```python
from build123d import *

# Parameters (mm, degrees)
SKETCH_1_R          = 6
EXTRUDE_1_DEPTH     = 5
SKETCH_7_R          = 7
EXTRUDE_6_DEPTH     = 1
EXTRUDE_2_DEPTH     = 13
CUT_EXTRUDE_1_DEPTH = 19


with BuildPart() as part:
    # 草图1 → 凸台-拉伸1 (new body)
    with BuildSketch(Plane.XY):
        Circle(SKETCH_1_R)
    extrude(amount=EXTRUDE_1_DEPTH)

    # 草图7 → 凸台-拉伸6 (add)
    with BuildSketch(Plane.XY.offset(5)):
        Circle(SKETCH_7_R)
    extrude(amount=-EXTRUDE_6_DEPTH)

    # 草图2 → 凸台-拉伸2 (add)
    with BuildSketch(Plane.XY.offset(5)):
        with BuildLine():
            ThreePointArc((4, 0), (1.414213562, 3.741657387), (-3, 2.645751311))
            Line((-3, 2.645751311), (-3, -2.645751311))
            ThreePointArc((-3, -2.645751311), (1.414213562, -3.741657387), (4, 0))
        make_face()
    extrude(amount=EXTRUDE_2_DEPTH)

    # 草图8 → 切除-拉伸1 (cut, through all)
    with BuildSketch(Plane.XY):
        with BuildLine():
            ThreePointArc((2.6, 0), (0.721110255, 2.497999199), (-2.2, 1.385640646))
            Line((-2.2, 1.385640646), (-2.2, -1.385640646))
            ThreePointArc((-2.2, -1.385640646), (0.721110255, -2.497999199), (2.6, 0))
        make_face()
    extrude(amount=CUT_EXTRUDE_1_DEPTH, mode=Mode.SUBTRACT)


solid = part.part
```
Design review of the part built by this model. Coordinates are the model's own, in mm. A direction names the side the tool comes from. Round coordinates to 2 decimals unless told otherwise and drop trailing zeros. Order: outer loops, then holes, each group sorted by start corner. A loop starts at its lowest first (then second) coordinate and runs counter-clockwise, first axis right, second up. Notation, with made-up numbers: (-28.5, 71) - (-19.5, 71) arc R25 ccw to (-19.5, 103) - close; hole circle Ø6 at (15.25, 47). An arc over 180 degrees is marked (long way). Return JSON: item names as keys, results as strings.
Q1. For pin 1 Ø4 at (y, z) = (-2, 14.5) entering from -X; pin 2 Ø1.5 at (y, z) = (-3, 5.5) entering from -X; pin 3 Ø1.5 at (x, z) = (-0.5, 2.5) entering from +Y, all flat-tipped, find the tip position at first contact; note any pin that passes through.
Computed values:
{"pin 1": "stops at x = -3", "pin 2": "stops at x = -6.56", "pin 3": "stops at y = 6"}
Q2. Consider section A-A on x = 0. Write out the cut boundary in (y, z), plus the area to 3 significant figures.
Computed values:
{"outline": "(-7, 4) - (-6, 4) - (-6, 0) - (-2.6, 0) - (-2.6, 18) - (-4, 18) - (-4, 5) - (-7, 5) - close; (2.6, 0) - (6, 0) - (6, 4) - (7, 4) - (7, 5) - (4, 5) - (4, 18) - (2.6, 18) - close", "area": "72.4 mm2"}
Q3. Wall thickness on L1, parallel to Z at x = -1, y = -5.75; L2, parallel to Y at x = 2, z = 11.5; L3, parallel to Z at x = 4.5, y = 5.25: over which ranges is each line inside the solid? List them lowest first. Write a range as [from, to].
Computed values:
{"L1": "z = [0, 5]", "L2": "y = [-3.46, -1.66], [1.66, 3.46]", "L3": "z = [4, 5]"}
Q4. Consider section D-D on x = -3.25. Write out the cut boundary in (y, z), plus the area to 3 significant figures.
Computed values:
{"outline": "(-6.2, 4) - (-5.04, 4) - (-5.04, 0) - (5.04, 0) - (5.04, 4) - (6.2, 4) - (6.2, 5) - (-6.2, 5) - close", "area": "52.7 mm2"}
Q5. Machinability: for faces 1 (the flat face through (-3.2, 0.1, 5)), 2 (the cylindrical face through (-6, 0, 2)), 3 (the flat face through (-3, 0, 11)), which of the approach directions +Z, -Z, +X, -X, +Y, -Y give a long, thin tool a straight path to every point of the face, cutting with its end or side? Answer none if there is none.
Computed values:
{"face 1": "+Z", "face 2": "-Z", "face 3": "+Z, -X, +Y, -Y"}
Q6. Consider section B-B on y = 2. Write out the cut boundary in (x, z).
Computed values:
{"outline": "(-6.71, 4) - (-5.66, 4) - (-5.66, 0) - (-1.66, 0) - (-1.66, 18) - (-3, 18) - (-3, 5) - (-6.71, 5) - close; (1.66, 0) - (5.66, 0) - (5.66, 4) - (6.71, 4) - (6.71, 5) - (3.46, 5) - (3.46, 18) - (1.66, 18) - close"}
Q7. The part is to be moulded in two halves that separate along Y. For faces 4 (the flat face through (2, -2, 18)), 5 (the flat face through (-2.2, 0, 9)), 6 (the cylindrical face through (6.466, -2.681, 4.507)), say which applies: pulls with the +Y half, pulls with the -Y half, needs draft (parallel to the pull), parting line crosses it, or undercut.
Computed values:
{"face 4": "needs draft", "face 5": "undercut", "face 6": "parting line crosses it"}
Q8. Consider section C-C on z = 15.5. Write out the cut boundary in (x, y), plus the area to 3 significant figures.
Computed values:
{"outline": "(-3, -2.65) arc R4 ccw (long way) to (-3, 2.65) - close; hole (-2.2, -1.39) arc R2.6 ccw (long way) to (-2.2, 1.39) - close", "area": "26.2 mm2"}
